from build123d import *

# Parameters (mm, degrees)
F0_R     = 279.4
F0_R_2   = 275.209
F1_DEPTH = 914.4
F2_W     = 327.650912
F2_H     = 123.030126
F3_DEPTH = 279.401
F4_R     = 2.070551
F5_DEPTH = 914.4


with BuildPart() as f1:
    # F0 (on Top) → F1 (new body)
    with BuildSketch(Plane.XY):
        Circle(F0_R)
        Circle(F0_R_2, mode=Mode.SUBTRACT)
    extrude(amount=F1_DEPTH)

    # F2 (on Front) → F3 (cut, through all)
    with BuildSketch(Plane.XZ):
        with Locations((-13.302971, 676.583201)):
            Rectangle(F2_W, F2_H)
    extrude(amount=-F3_DEPTH, mode=Mode.SUBTRACT)

    # F4 (on Top) → F5 (join)
    with BuildSketch(Plane.XY):
        with Locations((277.640581, 0)):
            Circle(F4_R)
    extrude(amount=F5_DEPTH)


solid = f1.part
Geometry check sheet. Reference: the model listing, model coordinates, mm. Coordinates: 2 decimals unless noted, no trailing zeros. Order: outer loops, then holes, each group sorted by start corner. A loop starts at its lowest first (then second) coordinate and runs counter-clockwise, first axis right, second up. Notation, with made-up numbers: M -7.75,18 L 46.25,18 A6 ccw 46.25,29 Z; hole C -22.5,21 d11. An arc over 180 degrees is marked long. Use CSV: the item, a comma, the result in double quotes.
Item 1: Cross-section at B-B on y = 97.5. Record the cut outline in (x, z), then the cut area to 3 significant figures.
Returned:
outline,"M -261.84,0 L -257.36,0 L -257.36,914.4 L -261.84,914.4 Z; M 257.36,0 L 261.84,0 L 261.84,914.4 L 257.36,914.4 Z"
area,"8,190 mm2"
Item 2: Cross-section at C-C on x = -195. Record the cut outline in (y, z), then the cut area to 3 significant figures.
Returned:
outline,"M -200.1,0 L -194.2,0 L -194.2,914.4 L -200.1,914.4 Z; M 194.2,0 L 200.1,0 L 200.1,914.4 L 194.2,914.4 Z"
area,"10,800 mm2"
Item 3: Mould release check, pull along Z, two halves, no side actions. Record for faces 1 (the flat face through (268.1, 63.4, 0)), 2 (the flat face through (268.1, 63.4, 914.4)), 3 (the flat face through (-14.1, 275.4, 738.098)), 4 (the flat face through (-14.1, 275.4, 615.068)): pulls with the +Z half, pulls with the -Z half, needs draft (parallel to the pull), parting line crosses it, or undercut.
Returned:
face 1,"pulls with the -Z half"
face 2,"pulls with the +Z half"
face 3,"undercut"
face 4,"undercut"
Item 4: Cross-section at D-D on x = -133.5. Record the cut outline in (y, z).
Returned:
outline,"M -245.44,0 L -240.66,0 L -240.66,914.4 L -245.44,914.4 Z; M 240.66,0 L 245.44,0 L 245.44,615.07 L 240.66,615.07 Z; M 240.66,738.1 L 245.44,738.1 L 245.44,914.4 L 240.66,914.4 Z"
Item 5: Cross-section at A-A on x = 0. Record the cut outline in (y, z).
Returned:
outline,"M -279.4,0 L -275.21,0 L -275.21,914.4 L -279.4,914.4 Z; M 275.21,0 L 279.4,0 L 279.4,615.07 L 275.21,615.07 Z; M 275.21,738.1 L 279.4,738.1 L 279.4,914.4 L 275.21,914.4 Z"
Item 6: Gauge pin test, flat ends, axial feed: pin 1 Ø6 at (y, z) = (214, 683.5) entering from +X; pin 2 Ø2 at (x, z) = (-179, 484) entering from +Y; pin 3 Ø5.5 at (y, z) = (233, 678) entering from -X. Record the tip position at first contact, or that the pin passes through.
Returned:
pin 1,"stops at x = 183.15"
pin 2,"stops at y = 215.36"
pin 3,"stops at x = 150.52"
Item 7: Thickness scan on line 1 along Y through (x, z) = (0, 241.5); line 2 along X through (y, z) = (-48, 612.5); line 3 along Y through (x, z) = (217, 865). Record the ranges inside material, lowest first.
Returned:
line 1,"y = -279.4 to -275.21, 275.21 to 279.4"
line 2,"x = -275.25 to -270.99, 270.99 to 275.25"
line 3,"y = -176 to -169.27, 169.27 to 176"
